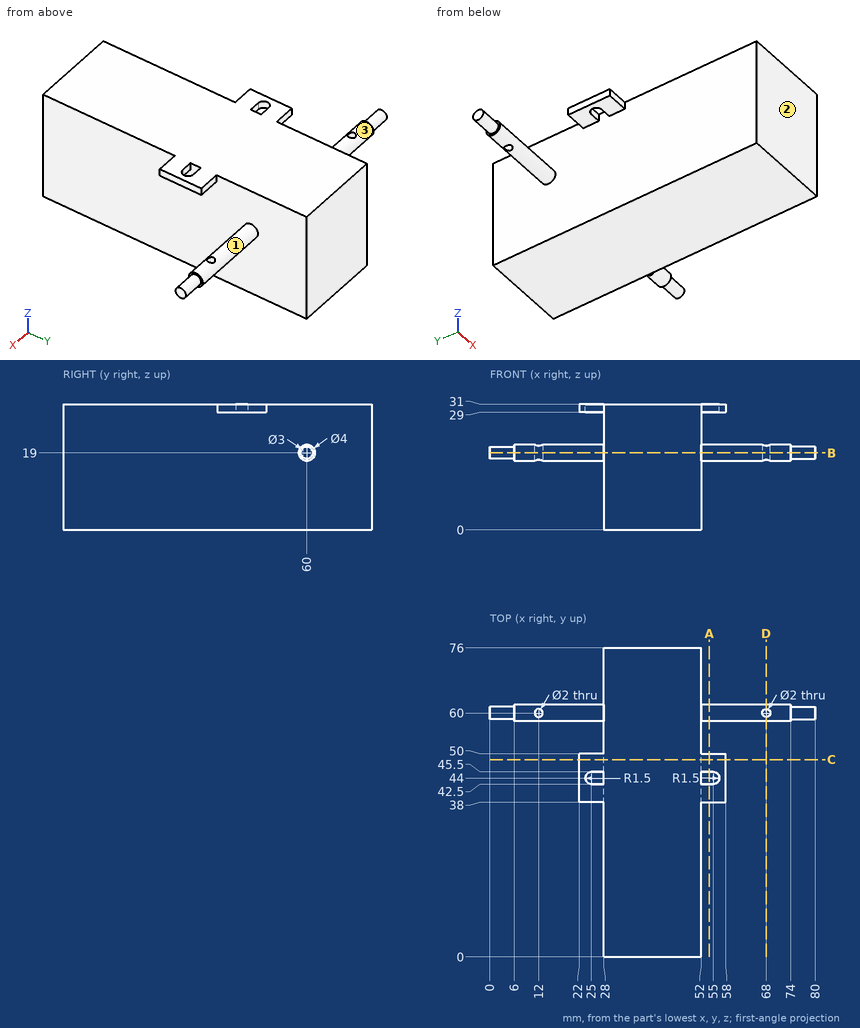
Print and shaded views of the part. All mm, measured from the part's lowest x, y and z. A direction names the side the tool comes from. Round coordinates to 2 decimals unless told otherwise and drop trailing zeros. Write each loop counter-clockwise with the first axis right and the second up, starting at its lowest first coordinate (ties: lowest second). Pieces come first, ordered by that corner, then holes. Notation, with made-up numbers: (87, 60) - (138, 60) arc R15 cw to (138, 70) - close; hole circle Ø1 at (26, 69.5). An arc over 180 degrees is marked (long way). Use CSV: the item, a comma, the result in double quotes. Start each with the question number.
Item 1: Tool access for the marked faces 1, 2 and 3: list every direction of +Z, -Z, +X, -X, +Y, -Y with a clear straight run to the whole face (end or side of a thin tool).
Item 2: Band-saw the part on D-D (x = 68). Write the cut outline in (y, z).
Item 3: Band-saw the part on A-A (x = 54). Write the cut outline in (y, z).
Item 4: Band-saw the part on C-C (y = 48.5). Write the cut outline in (x, z).
Item 5: Band-saw the part on B-B (z = 19). Write the cut outline in (x, y), and give its area (3 significant figures).
Item 6: Pin check, flat tips, straight feed: P1, Ø2.5, axis at x = 12, y = 60, coming from the -Z side; P2, Ø2, axis at y = 34.5, z = 8, coming from the -X side; P3, Ø1, axis at y = 42.5, z = 30, coming from the +X side. Stop position of each tip, or through.
Item 7: Drill centre lines: L1, parallel to X at y = 60, z = 18.55; L2, parallel to Y at x = 68, z = 18.85; L3, parallel to X at y = 51, z = 25. Where is each one in solid material? Low to high. Write a range as [from, to].
Checked values:
1,face 1,"+X"
1,face 2,"+Z, -Z, +X, -X, -Y"
1,face 3,"-X"
2,outline,"(59, 17.27) - (59, 20.73) arc R2 ccw to start; (61, 17.27) arc R2 ccw to (61, 20.73) - close"
3,outline,"(38, 29) - (42.5, 29) - (42.5, 31) - (38, 31) - close; (45.5, 29) - (50, 29) - (50, 31) - (45.5, 31) - close; circle Ø4 at (60, 19)"
4,outline,"(22, 29) - (28, 29) - (28, 0) - (52, 0) - (52, 29) - (58, 29) - (58, 31) - (22, 31) - close"
5,outline,"(0, 58.5) - (6, 58.5) - (6, 58) - (28, 58) - (28, 0) - (52, 0) - (52, 58) - (74, 58) - (74, 58.5) - (80, 58.5) - (80, 61.5) - (74, 61.5) - (74, 62) - (52, 62) - (52, 76) - (28, 76) - (28, 62) - (6, 62) - (6, 61.5) - (0, 61.5) - close; hole circle Ø2 at (12, 60); hole circle Ø2 at (68, 60)"
5,area,"2,030 mm²"
6,P1,"stops at z = 17"
6,P2,"stops at x = 28"
6,P3,"stops at x = 58"
7,L1,"x = [0, 11], [13, 67], [69, 80]"
7,L2,"y = [58.01, 59], [61, 61.99]"
7,L3,"x = [28, 52]"
